Drawing for the job (mm, zero at the part's lowest x, y, z). A direction names the side the tool comes from. Round coordinates to 2 decimals unless told otherwise and drop trailing zeros. Loops run counter-clockwise (first coordinate to the right, second up) from the corner with the lowest first, then second, coordinate; pieces in that order, holes last. Notation, with made-up numbers: (34.25, 14) -> (83.25, 14) arc R19 ccw to (83.25, 22) -> close; hole circle Ø4 at (-16, 43). An arc over 180 degrees is marked (long way). Put each result on its own line as item: value. Start each with the question number.
Item 1: Cut at A-A, the plane z = 7.5. List the corners of the cut face in (x, y) (3 decimals), plus the area to 3 significant figures.
Item 2: Cut at B-B, the plane z = 2. List the corners of the cut face in (x, y) (3 decimals).
Item 3: Drill centre lines: probe 1 along Z at (x, y) = (9, 3.5); probe 2 along Z at (x, y) = (10.75, 4.25); probe 3 along Y at (x, z) = (6, 5.5). Where is each one in solid material? Low to high. Write a range as [from, to].
Item 4: Pull direction Z, two halves, no side cores. Call the marked faces 1, 2 and 3: +Z half, -Z half, draft (parallel to the pull), parting line (faces both ways), or undercut.
Item 5: Tool access for the marked faces 4, 5 and 6: list every direction of +Z, -Z, +X, -X, +Y, -Y with a clear straight run to the whole face (end or side of a thin tool).
Item 6: Flat gauge pins, fed straight in: pin 1 Ø5 at (x, z) = (9, 8.5) entering from +Y; pin 2 Ø1.5 at (y, z) = (10, 2) entering from -X; pin 3 Ø1 at (x, z) = (9, 9.5) entering from -Y. Where does each tip first touch, or does it go through?
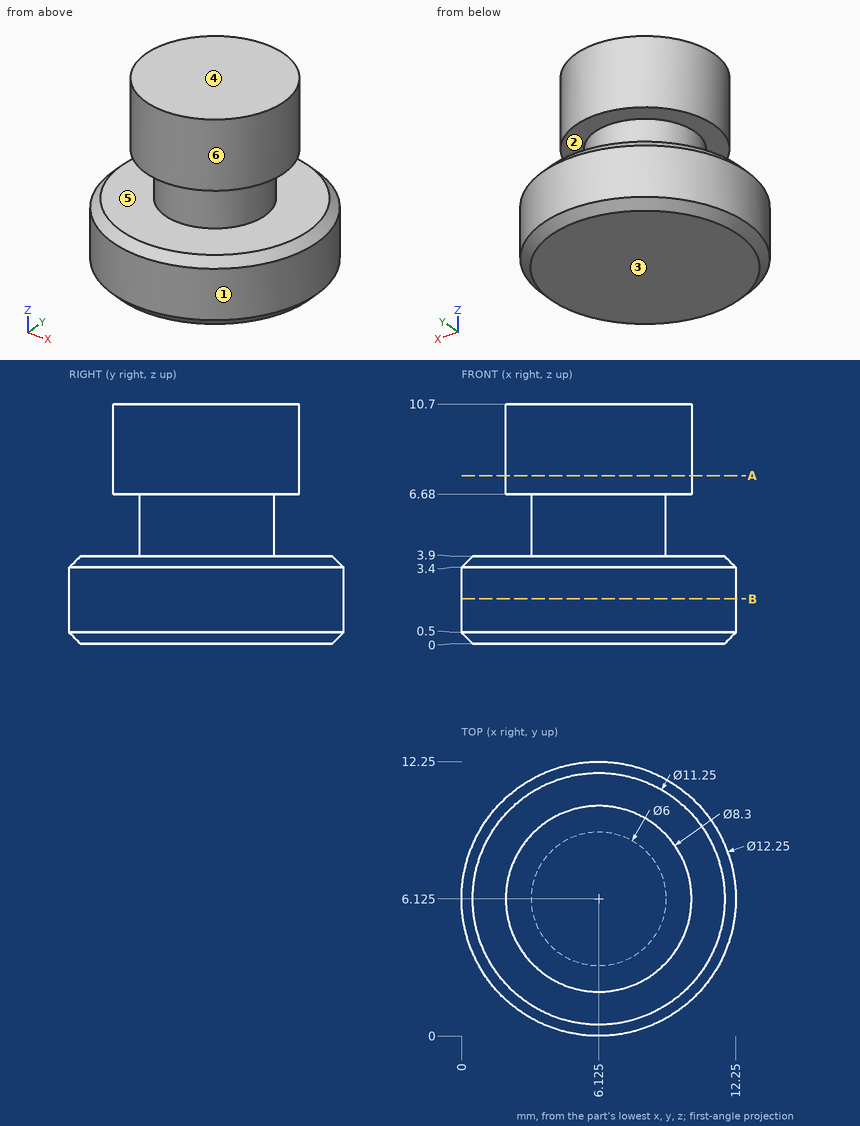
Reply:
1. outline: circle Ø8.3 at (6.125, 6.125)
1. area: 54.1 mm^2
2. outline: circle Ø12.25 at (6.125, 6.125)
3. probe 1: z = [0, 3.9], [6.68, 10.7]
3. probe 2: z = [0, 3.9]
3. probe 3: y = [3.13, 9.12]
4. face 1: draft
4. face 2: undercut
4. face 3: -Z half
5. face 4: +Z, +X, -X, +Y, -Y
5. face 5: none
5. face 6: +Z
6. pin 1: stops at y = 10.26
6. pin 2: stops at x = 0.86
6. pin 3: stops at y = 2.72
